Input: part model. Units: mm. Frame: model coordinates. A direction names the side the tool comes from. Give positions to 0.01 mm unless a question says otherwise; leave off trailing zeros. Order: outer loops, then holes, each group sorted by start corner. A loop starts at its lowest first (then second) coordinate and runs counter-clockwise, first axis right, second up. Notation, with made-up numbers: M -28.5,-15 L -19.5,-15 A38 cw -19.5,23 Z; hole C 63.5,39 d4. An arc over 180 degrees is marked long. Use a Markdown table: item, result.
from build123d import *

# Parameters (mm, degrees)
F0_R     = 50
F1_DEPTH = 10.5
F2_R     = 22.3
F3_DEPTH = 9.4
F6_D     = 8.1
F7_R     = 10.115
F8_DEPTH = 25


with BuildPart() as f1:
    # F0 (on Top) → F1 (new body)
    with BuildSketch(Plane.XY):
        Circle(F0_R)
    extrude(amount=F1_DEPTH)

    # F2 (on face) → F3 (join)
    with BuildSketch(Plane.XY.offset(10.5)):
        Circle(F2_R)
    extrude(amount=F3_DEPTH)

    # F6 (through all)
    with Locations(Plane.XY.offset(10.5)):
        with Locations((0, 43.061581), (30.449136, 30.449136), (43.061581, 0), (30.449136, -30.449136), (0, -43.061581), (-30.449136, -30.449136), (-43.061581, 0), (-30.449136, 30.449136)):
            Hole(F6_D / 2)

    # F7 (on face) → F8 (cut)
    with BuildSketch(Plane.XY.offset(19.9)):
        Circle(F7_R)
    extrude(amount=-F8_DEPTH, mode=Mode.SUBTRACT)


solid = f1.part
1) Mould query, pull axis X, two halves, no side actions, for faces 3 (the face through (0.88, 39.11, 5.18)), 4 (the face through (-0.7, -10.4, 0)), 5 (the face through (47.69, 15.02, 5.18)). Classes: released by +X, released by -X, zero draft, split by the parting line, or undercut.
Response values:
| item | result |
|---|---|
| face 3 | undercut |
| face 4 | zero draft |
| face 5 | split by the parting line |
2) Material intervals for line 1 (Y direction, x = 0, z = 5.5) (3 decimals); line 2 (Y direction, x = 0, z = 14) (3 decimals); line 3 (Z direction, x = -1.5, y = 37.5), sorted ascending. Write a range as from..to.
Response values:
| item | result |
|---|---|
| line 1 | y = -50..-47.112, -39.012..-10.115, 10.115..39.012, 47.112..50 |
| line 2 | y = -22.3..-10.115, 10.115..22.3 |
| line 3 | z = 0..10.5 |
3) Reachability of faces 1 (the face through (-23, 1, 10.5)), 2 (the face through (0.878, -47.015, 5.177)) from +Z, -Z, +X, -X, +Y, -Y: full face, straight path, thin tool, end or side. Return the list, or none.
Response values:
| item | result |
|---|---|
| face 1 | +Z |
| face 2 | +Z, -Z |
4) Cut plane D-D on x = -32.5. Return loops of the section in (y, z).
Response values:
| item | result |
|---|---|
| outline | M -38,0 L -33.94,0 L -33.94,10.5 L -38,10.5 Z; M -26.96,0 L 26.96,0 L 26.96,10.5 L -26.96,10.5 Z; M 33.94,0 L 38,0 L 38,10.5 L 33.94,10.5 Z |
5) First-contact query: pin 1 Ø1 at (x, y) = (11.5, -24.5) entering from +Z; pin 2 Ø2 at (x, z) = (-30, 9) entering from -Y; pin 3 Ø8 at (y, z) = (-19.5, 12.5) entering from +X. Flat tips, straight axial feed; report the tip coordinate or a pass-through.
Response values:
| item | result |
|---|---|
| pin 1 | stops at z = 10.5 |
| pin 2 | stops at y = -40.73 |
| pin 3 | stops at x = 47.36 |
6) Cut plane C-C on z = 7. State how many separate pieces and enclosed holes the cut face has, and give its area (3 significant figures).
Response values:
| item | result |
|---|---|
| separate pieces | 1 |
| enclosed holes | 9 |
| area | 7,120 mm² |
7) Cut plane A-A on x = 0. Return loops of the section in (y, z) (3 decimals), and give its area (3 significant figures).
Response values:
| item | result |
|---|---|
| outline | M -50,0 L -47.112,0 L -47.112,10.5 L -50,10.5 Z; M -39.012,0 L -10.115,0 L -10.115,19.9 L -22.3,19.9 L -22.3,10.5 L -39.012,10.5 Z; M 10.115,0 L 39.012,0 L 39.012,10.5 L 22.3,10.5 L 22.3,19.9 L 10.115,19.9 Z; M 47.112,0 L 50,0 L 50,10.5 L 47.112,10.5 Z |
| area | 897 mm² |
